Design review of the part built by this model. Coordinates are the model's own, in mm. A direction names the side the tool comes from. Coordinates: 2 decimals unless noted, no trailing zeros. Loops run counter-clockwise (first coordinate to the right, second up) from the corner with the lowest first, then second, coordinate; pieces in that order, holes last. Notation, with made-up numbers: M 68.5,-25.5 L 103.5,-25.5 A22 cw 103.5,10.5 Z; hole C 33.25,-21 d8. An arc over 180 degrees is marked long. Write item = value, one per line. Start each with the question number.
from build123d import *

# Parameters (mm, degrees)
SKETCH2_R           = 1.5
BOSS_EXTRUDE1_DEPTH = 7
BOSS_EXTRUDE2_DEPTH = 9
FILLET3_R           = 1
CUT_EXTRUDE1_DEPTH  = 10.517452338


with BuildPart() as part:
    # Sketch2 → Boss-Extrude1 (new body)
    with BuildSketch(Plane(origin=(0, 0, 0), x_dir=(1, 0, 0), z_dir=(0, 1, 0))):
        with BuildLine():
            Line((-12.939762178, 2.094266176), (-24.821781773, 3.29179515))
            ThreePointArc((-24.821781773, 3.29179515), (-30.987291256, -0.071668068), (-24.821747911, -3.435069212))
            Line((-24.821747911, -3.435069212), (-12.987160246, -2.166440487))
            ThreePointArc((-12.987160246, -2.166440487), (-10.8566751, -0.059524017), (-12.939762178, 2.094266176))
        make_face()
        with Locations((-26.987114413, 0)):
            Circle(SKETCH2_R, mode=Mode.SUBTRACT)
    extrude(amount=BOSS_EXTRUDE1_DEPTH)

    # Sketch2_3 → Boss-Extrude2 (add)
    with BuildSketch(Plane(origin=(0, 0, 0), x_dir=(1, 0, 0), z_dir=(0, 1, 0))):
        with BuildLine():
            Line((-26.987114411, -4.57148105), (-25.802758185, -4.412822706))
            ThreePointArc((-25.802758185, -4.412822706), (-24.779096258, -3.992509307), (-23.88896632, -3.335078105))
            Line((-23.88896632, -3.335078105), (-24.821747911, -3.435069212))
            ThreePointArc((-24.821747911, -3.435069212), (-30.987291256, -0.071668068), (-24.821781773, 3.29179515))
            Line((-24.821781773, 3.29179515), (-23.896053235, 3.198495628))
            ThreePointArc((-23.896053235, 3.198495628), (-24.802641315, 3.862379952), (-25.845447528, 4.2809484))
            Line((-25.845447528, 4.2809484), (-26.987114411, 4.428185187))
            ThreePointArc((-26.987114411, 4.428185187), (-31.48694753, -0.071647931), (-26.987114411, -4.57148105))
        make_face()
        with BuildLine():
            Line((-25.802758185, -4.412822706), (-12.637077878, -2.649126119))
            ThreePointArc((-12.637077878, -2.649126119), (-13.508046926, -2.620506326), (-14.322115833, -2.309543319))
            Line((-14.322115833, -2.309543319), (-23.88896632, -3.335078105))
            ThreePointArc((-23.88896632, -3.335078105), (-24.779096258, -3.992509307), (-25.802758185, -4.412822706))
        make_face()
        with BuildLine():
            ThreePointArc((-14.328363864, 2.234216353), (-13.517942982, 2.546845227), (-12.649914094, 2.579166576))
            Line((-12.649914094, 2.579166576), (-25.845447528, 4.2809484))
            ThreePointArc((-25.845447528, 4.2809484), (-24.802641315, 3.862379952), (-23.896053235, 3.198495628))
            Line((-23.896053235, 3.198495628), (-14.328363864, 2.234216353))
        make_face()
        with BuildLine():
            ThreePointArc((-12.637077878, -2.649126119), (-11.057896416, -1.833001646), (-10.355629468, -0.2))
            Line((-10.355629468, -0.2), (-10.371987074, 0.3))
            ThreePointArc((-10.371987074, 0.3), (-11.122262116, 1.828060363), (-12.649914094, 2.579166576))
            ThreePointArc((-12.649914094, 2.579166576), (-13.517942982, 2.546845227), (-14.328363864, 2.234216353))
            Line((-14.328363864, 2.234216353), (-12.939762178, 2.094266176))
            ThreePointArc((-12.939762178, 2.094266176), (-11.463920967, 1.453898193), (-10.856543276, -0.035823517))
            ThreePointArc((-10.856543276, -0.035823517), (-11.480586539, -1.542397225), (-12.987160246, -2.166440487))
            Line((-12.987160246, -2.166440487), (-14.322115833, -2.309543319))
            ThreePointArc((-14.322115833, -2.309543319), (-13.508046926, -2.620506326), (-12.637077878, -2.649126119))
        make_face()
        with BuildLine():
            ThreePointArc((-12.649914094, 2.579166576), (-11.122262116, 1.828060363), (-10.371987074, 0.3))
            Line((-10.371987074, 0.3), (-5.980159731, 0.3))
            Line((-5.980159731, 0.3), (-5.980159731, 1.71899167))
            Line((-5.980159731, 1.71899167), (-12.649914094, 2.579166576))
        make_face()
        with BuildLine():
            Line((-5.980021524, -1.757335699), (-5.980297938, -0.2))
            Line((-5.980297938, -0.2), (-10.355629468, -0.2))
            ThreePointArc((-10.355629468, -0.2), (-11.057896416, -1.833001646), (-12.637077878, -2.649126119))
            Line((-12.637077878, -2.649126119), (-5.980021524, -1.757335699))
        make_face()
    extrude(amount=BOSS_EXTRUDE2_DEPTH)

    # Fillet3
    fillet3_edges = [part.edges().sort_by_distance(p)[0] for p in [
        (-5.980159731, 4.5, -0.3),
        (-5.980297938, 4.5, 0.2),
    ]]
    fillet(fillet3_edges, radius=FILLET3_R)

    # Sketch3 → Cut-Extrude1 (cut, through all)
    with BuildSketch(Plane(origin=(0.125841463, 0, 0.939384066), x_dir=(0.991146125, 0, -0.132775595), z_dir=(0.132775595, 0, 0.991146125))):
        with BuildLine():
            Line((-8.079177289, 3.2), (-10.730603596, 3.2))
            ThreePointArc((-10.730603596, 3.2), (-12.030603596, 4.5), (-10.730603596, 5.8))
            Line((-10.730603596, 5.8), (-8.079177289, 5.8))
            ThreePointArc((-8.079177289, 5.8), (-6.779177289, 4.5), (-8.079177289, 3.2))
        make_face()
    extrude(amount=-CUT_EXTRUDE1_DEPTH, mode=Mode.SUBTRACT)


solid = part.part
Q1. Clearance check with flat-ended pins moving along their axes: P1, Ø2.5, axis at x = -19.5, z = 0, coming from the +Y side; P2, Ø2.5, axis at x = -9.5, y = 2, coming from the +Z side; P3, Ø1.7, axis at x = -8.5, y = 6.5, coming from the +Z side. State where each tip first meets the part, or that it passes through.
Q2. Add section D-D on x = -16.75. State the section outline as (y, z) points.
Q3. To check wall thickness, follow line 1 (Y direction, x = -9.5, z = -1.25); line 2 (Y direction, x = -19.5, z = 1); line 3 (X direction, y = 4.5, z = 0.5). State the ranges of each line that lie inside material, in increasing order. Write a range as from..to.
Q4. Add section B-B on x = -9.5. State the section outline as (y, z) points, plus the area to 3 significant figures.
Q5. Mouldability with a two-part tool opening along Z and no side actions: class faces 6 (the face through (-21, 7, 0)), 7 (the face through (-6, 5, 1)), 8 (the face through (-18, 9, 3)), 9 (the face through (-6.713, 4.529, 0.946)) as released by +Z, released by -Z, zero draft, split by the parting line, or undercut.
Q6. Add section A-A on y = 6.25. State the section outline as (x, z) points, plus the area to 3 significant figures.
Q7. Add section C-C on x = -21. State the section outline as (y, z) points.
Q8. For faces 1 (the face through (-7, 4.5, -1.2)), 2 (the face through (-12.14, 4.47, -0.01)), 3 (the face through (-30.985, 7.986, 0.192)), 4 (the face through (-6.281, 4.563, -0.585)), 5 (the face through (-28.486, 3.451, -0.066)), list the 3-axis set-ups (+Z, -Z, +X, -X, +Y, -Y) from which the entire face can be reached by the end or side of a thin tool; tool diameter is ignored.
Values follow:
q1.P1 = 7
q1.P2 = 2.4
q1.P3 = 2.21
q2.outline = M 0,-3.11 L 9,-3.11 L 9,-2.48 L 7,-2.48 L 7,2.57 L 9,2.57 L 9,3.2 L 0,3.2 Z
q3.line_1 = 0..3.2, 5.8..9
q3.line_2 = 0..7
q3.line_3 = -31.47..-28.4, -25.57..-12.07, -6.77..-6.27
q4.outline = M 0,-2.17 L 3.2,-2.17 L 3.2,-0.3 L 0,-0.3 Z; M 0,0.2 L 3.2,0.2 L 3.2,2.23 L 0,2.23 Z; M 5.8,-2.17 L 9,-2.17 L 9,-0.3 L 5.8,-0.3 Z; M 5.8,0.2 L 9,0.2 L 9,2.23 L 5.8,2.23 Z
q4.area = 25.0 mm2
q5.face_6 = undercut
q5.face_7 = undercut
q5.face_8 = zero draft
q5.face_9 = released by +Z
q6.outline = M -26.99,-4.43 L -5.98,-1.72 L -5.98,-1.3 A1 ccw -6.98,-0.3 L -10.37,-0.3 L -10.36,0.2 L -6.98,0.2 A1 ccw -5.98,1.2 L -5.98,1.76 L -26.99,4.57 A4.5 ccw Z; hole C -26.99,0 d3
q6.area = 153 mm2
q7.outline = M 0,-3.66 L 9,-3.66 L 9,-2.91 L 7,-2.91 L 7,3.03 L 9,3.03 L 9,3.77 L 0,3.77 Z
q8.face_1 = +Z
q8.face_2 = -Z
q8.face_3 = +Y
q8.face_4 = +X, +Y, -Y
q8.face_5 = +Y, -Y
